Here's the drawing with two shaded views (mm, measured from the low corner). I have some questions. Coordinates: 2 decimals unless noted, no trailing zeros. Write each loop counter-clockwise with the first axis right and the second up, starting at its lowest first coordinate (ties: lowest second). Pieces come first, ordered by that corner, then holes.
Item 1: I'm going to push flat-ended pins straight in: pin 1 Ø9 at (x, z) = (50, 70) entering from +Y; pin 2 Ø1 at (y, z) = (1, 34) entering from -X; pin 3 Ø1.5 at (x, y) = (8.5, 2.5) entering from -Z; pin 4 Ø5 at (x, z) = (50, 10) entering from -Y. Where does each tip first touch, or does it pass through?
Item 2: If we section it at C-C (x = 55): Please give me the cut outline in (y, z).
Item 3: If we section it at A-A (y = 3.9): Please give me the cut outline in (x, z).
Item 4: If I drill on line 1 (X direction, y = 3.5, z = 10); line 2 (X direction, y = 2.3, z = 7); line 3 (Z direction, x = 53, y = 2.8), over which ranges is the centre line in solid material (lowest first)?
Item 5: If we section it at B-B (z = 33): Please give me the cut outline in (x, y).
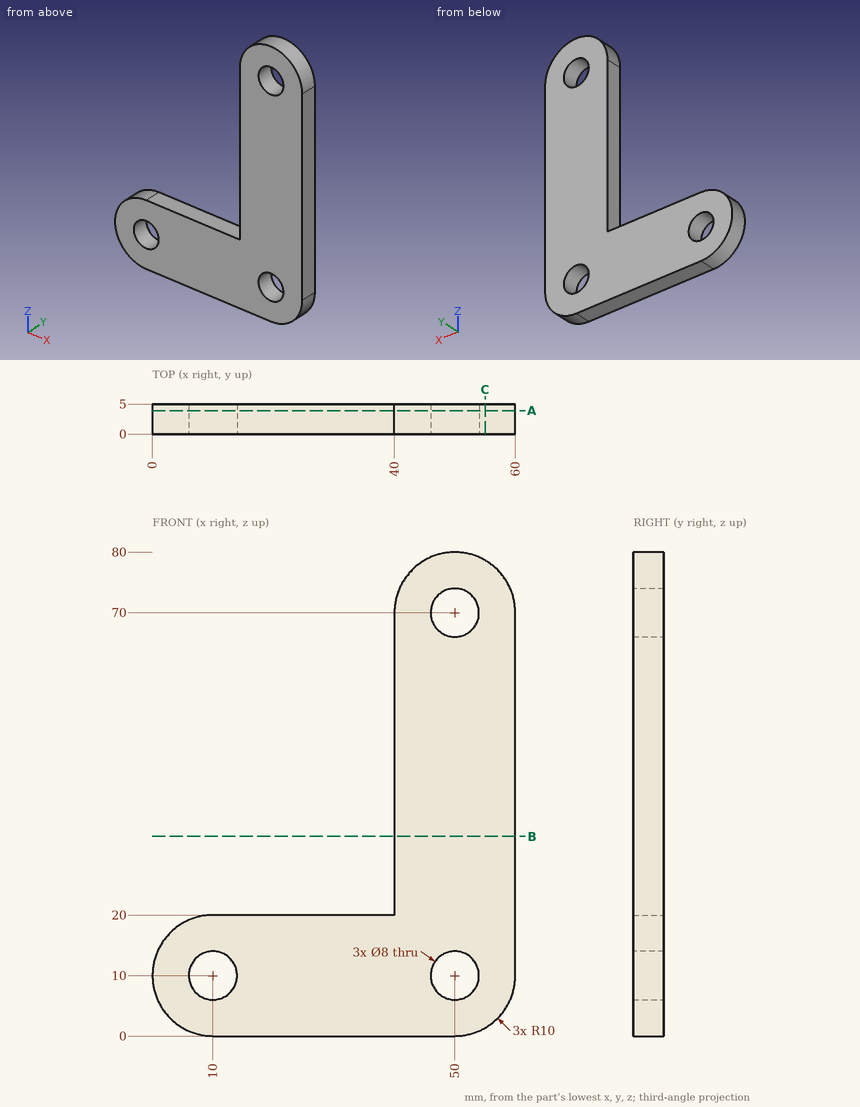
Answer list:
1. pin 1: stops at y = 5
1. pin 2: stops at x = 40
1. pin 3: stops at z = 0.03
1. pin 4: passes through
2. outline: (0, 1.34) - (5, 1.34) - (5, 78.66) - (0, 78.66) - close
3. outline: (10, 0) - (50, 0) arc R10 ccw to (60, 10) - (60, 70) arc R10 ccw to (40, 70) - (40, 20) - (10, 20) arc R10 ccw to start; hole circle Ø8 at (10, 10); hole circle Ø8 at (50, 10); hole circle Ø8 at (50, 70)
4. line 1: x = 0 to 6, 14 to 46, 54 to 60
4. line 2: x = 0.46 to 7.35, 12.65 to 47.35, 52.65 to 59.54
4. line 3: z = 0.46 to 7.35, 12.65 to 67.35, 72.65 to 79.54
5. outline: (40, 0) - (60, 0) - (60, 5) - (40, 5) - close
